from build123d import *

# Parameters (mm, degrees)
F0_W     = 60
F0_H     = 60
F1_DEPTH = 2
F2_W     = 50
F2_H     = 50
F3_DEPTH = 10
F4_R     = 2


with BuildPart() as f1:
    # F0 (on Front) → F1 (new body)
    with BuildSketch(Plane.XZ):
        Rectangle(F0_W, F0_H)
    extrude(amount=F1_DEPTH)

    # F2 (on face) → F3 (join)
    with BuildSketch(Plane.XZ.offset(2)):
        Rectangle(F2_W, F2_H)
    extrude(amount=F3_DEPTH)

    # F4
    f4_edges = [f1.edges().sort_by_distance(p)[0] for p in [
        (30, -1, -30),
        (30, -1, 30),
        (-30, -1, 30),
        (-30, -1, -30),
    ]]
    fillet(f4_edges, radius=F4_R)


solid = f1.part
Can you work these out from the model? Positions are in its coordinate system, mm. A direction names the side the tool comes from. Round coordinates to 2 decimals unless told otherwise and drop trailing zeros. Order: outer loops, then holes, each group sorted by start corner. A loop starts at its lowest first (then second) coordinate and runs counter-clockwise, first axis right, second up. Notation, with made-up numbers: M 67,61.5 L 125,61.5 A13 cw 125,76.5 Z; hole C 39,18.25 d3. An arc over 180 degrees is marked long. Use a Markdown table: item, result.
1) I'm going to push flat-ended pins straight in: P1, Ø1.5, axis at y = -8.5, z = 3, coming from the +X side; P2, Ø4, axis at x = 24, z = -12, coming from the +Y side; P3, Ø1.5, axis at x = 12.5, y = -5.5, coming from the +Z side; P4, Ø5, axis at y = -9.5, z = -9, coming from the -X side. Where does each tip first touch, or does it pass through?
Geometry says:
| item | result |
|---|---|
| P1 | stops at x = 25 |
| P2 | stops at y = 0 |
| P3 | stops at z = 25 |
| P4 | stops at x = -25 |
2) Imagine slicing it at A-A (x = -17). List the corners of the cut face in (y, z) for me, then the cut area to 3 significant figures.
Geometry says:
| item | result |
|---|---|
| outline | M -12,-25 L -2,-25 L -2,-30 L 0,-30 L 0,30 L -2,30 L -2,25 L -12,25 Z |
| area | 620 mm² |
3) If we mould it in two halves opening along X, with no side actions, what happens to faces 5 (the face through (-25, -7, 0)), 6 (the face through (29.4, -1.01, 29.43)), 7 (the face through (-27, -2, 0))? For each: +X half, -X half, draft (parallel to the pull), parting line (faces both ways), or undercut.
Geometry says:
| item | result |
|---|---|
| face 5 | -X half |
| face 6 | +X half |
| face 7 | draft |
4) Imagine slicing it at B-B (z = 5.5). List the corners of the cut face in (x, y) for me.
Geometry says:
| item | result |
|---|---|
| outline | M -30,-2 L -25,-2 L -25,-12 L 25,-12 L 25,-2 L 30,-2 L 30,0 L -30,0 Z |
5) Imagine slicing it at C-C (y = -4.25). List the corners of the cut face in (x, z) for me, then the cut area to 3 significant figures.
Geometry says:
| item | result |
|---|---|
| outline | M -25,-25 L 25,-25 L 25,25 L -25,25 Z |
| area | 2,500 mm² |
6) On a 3-axis mill with a long thin cutter (end or side, diameter ignored), from which of +Z, -Z, +X, -X, +Y, -Y can I reach the whole of each face in a straight line? I mean faces 1 (the face through (0, -7, 25)), 2 (the face through (-30, -1, 0)), 3 (the face through (0, -7, -25)), 4 (the face through (25, -7, 0)). Say none if no direction works.
Geometry says:
| item | result |
|---|---|
| face 1 | +Z, +X, -X, -Y |
| face 2 | +Z, -Z, -X, +Y, -Y |
| face 3 | -Z, +X, -X, -Y |
| face 4 | +Z, -Z, +X, -Y |
7) Imagine slicing it at D-D (x = 26). List the corners of the cut face in (y, z) for me.
Geometry says:
| item | result |
|---|---|
| outline | M -2,-30 L 0,-30 L 0,30 L -2,30 Z |
8) If I drill on line 1 along X through (y, z) = (-3.25, -17.5); line 2 along Y through (x, z) = (9, 27), over which ranges is the centre line in solid material (lowest first)?
Geometry says:
| item | result |
|---|---|
| line 1 | x = -25 to 25 |
| line 2 | y = -2 to 0 |
